The model under review builds one solid part; all positions refer to its coordinate system, in mm. A direction names the side the tool comes from. Give positions to 0.01 mm unless a question says otherwise; leave off trailing zeros. Loops run counter-clockwise (first coordinate to the right, second up) from the corner with the lowest first, then second, coordinate; pieces in that order, holes last. Notation, with made-up numbers: (89.5, -7) - (112.5, -7) arc R22 ccw to (112.5, 24) - close; hole circle Ø11 at (68.25, -27). An arc over 180 degrees is marked (long way). Answer as a JSON object with one key per item and string values.
from build123d import *

# Parameters (mm, degrees)
F0_R     = 26.9884014256
F1_DEPTH = 7
F2_R     = 32.0417466588
F2_R_2   = 26.9884014256
F3_DEPTH = 3
F4_R     = 11.1906834264
F5_DEPTH = 7
F6_R     = 4.0199304585
F7_DEPTH = 25
F9_DEPTH = 25
F10_SIZE = 5
F11_SIZE = 2


with BuildPart() as f1:
    # F0 (on Top) → F1 (new body)
    with BuildSketch(Plane.XY):
        Circle(F0_R)
    extrude(amount=F1_DEPTH)

    # F2 (on face) → F3 (join)
    with BuildSketch(Plane.XY.offset(7)):
        Circle(F2_R)
        Circle(F2_R_2, mode=Mode.SUBTRACT)
        Circle(F2_R_2)
    extrude(amount=F3_DEPTH)

    # F4 (on face) → F5 (cut)
    with BuildSketch(Plane.XY.offset(10)):
        Circle(F4_R)
    extrude(amount=-F5_DEPTH, mode=Mode.SUBTRACT)

    # F6 (on face) → F7 (cut)
    with BuildSketch(Plane.XY.offset(3)):
        Circle(F6_R)
    extrude(amount=-F7_DEPTH, mode=Mode.SUBTRACT)

    # F8 (on face) → F9 (cut)
    with BuildSketch(Plane.XY.offset(10)):
        with BuildLine():
            ThreePointArc((-15.0136980872, 1.4416950877), (-10.584772446, 10.7448688798), (-1.2161651409, 15.0336475058))
            Line((-1.2161651409, 15.0336475058), (-1.2161651409, 28.0388555672))
            ThreePointArc((-1.2161651409, 28.0388555672), (-19.7651192157, 19.9247720578), (-28.0281643074, 1.4416950877))
            Line((-28.0281643074, 1.4416950877), (-15.0136980872, 1.4416950877))
        make_face()
        with BuildLine():
            ThreePointArc((1.2975777549, 15.0268395529), (10.5846814228, 10.7449585461), (15.0056430278, 1.5232505708))
            Line((15.0056430278, 1.5232505708), (28.0238503219, 1.5232505708))
            ThreePointArc((28.0238503219, 1.5232505708), (19.7650570518, 19.9248337234), (1.2975777549, 28.0352059228))
            Line((1.2975777549, 28.0352059228), (1.2975777549, 15.0268395529))
        make_face()
        with BuildLine():
            ThreePointArc((15.0298348497, -1.262410143), (10.7403927, -10.5893144079), (1.4751854085, -15.0104444634))
            Line((1.4751854085, -15.0104444634), (1.4751854085, -28.0264215906))
            ThreePointArc((1.4751854085, -28.0264215906), (19.9202803133, -19.7696462135), (28.0368115127, -1.262410143))
            Line((28.0368115127, -1.262410143), (15.0298348497, -1.262410143))
        make_face()
        with BuildLine():
            ThreePointArc((-1.1481693356, -15.038993389), (-10.6271050963, -10.7030020205), (-15.0304418379, -1.2551625933))
            Line((-15.0304418379, -1.2551625933), (-28.0371369086, -1.2551625933))
            ThreePointArc((-28.0371369086, -1.2551625933), (-19.8072075166, -19.8829326197), (-1.1481693356, -28.0417222428))
            Line((-1.1481693356, -28.0417222428), (-1.1481693356, -15.038993389))
        make_face()
    extrude(amount=-F9_DEPTH, mode=Mode.SUBTRACT)

    # F10
    f10_edges = [f1.edges().sort_by_distance(p)[0] for p in [
        (-10.584772, 10.744869, 0),
        (10.584681, 10.744959, 0),
        (-10.627105, -10.703002, 0),
        (10.740393, -10.589314, 0),
    ]]
    chamfer(f10_edges, length=F10_SIZE)

    # F11
    f11_edges = [f1.edges().sort_by_distance(p)[0] for p in [
        (10.740393, -10.589314, 5),
        (-10.627105, -10.703002, 5),
        (10.584681, 10.744959, 5),
        (-10.584772, 10.744869, 5),
    ]]
    chamfer(f11_edges, length=F11_SIZE)


solid = f1.part
Q1. Consider section C-C, the plane z = 8.75. State the section outline as (x, y) points, plus the area to 3 significant figures.
Results:
{"outline": "circle Ø64.08 at (0, 0); hole (-28.04, -1.26) arc R28.07 ccw to (-1.15, -28.04) - (-1.15, -15.04) arc R15.08 cw to (-15.03, -1.26) - close; hole (-28.03, 1.44) - (-15.01, 1.44) arc R15.08 cw to (-1.22, 15.03) - (-1.22, 28.04) arc R28.07 ccw to start; hole circle Ø22.38 at (0, 0); hole (1.3, 15.03) arc R15.08 cw to (15.01, 1.52) - (28.02, 1.52) arc R28.07 ccw to (1.3, 28.04) - close; hole (1.48, -28.03) arc R28.07 ccw to (28.04, -1.26) - (15.03, -1.26) arc R15.08 cw to (1.48, -15.01) - close", "area": "1,210 mm^2"}
Q2. Clearance check with flat-ended pins moving along their axes: pin 1 Ø3 at (x, z) = (-11.5, 3.5) entering from +Y; pin 2 Ø1.5 at (x, z) = (-6.5, 8) entering from +Y; pin 3 Ø3 at (y, z) = (21, 6.5) entering from +X. State where each tip first meets the part, or that it passes through.
Results:
{"pin 1": "stops at y = 9.51", "pin 2": "stops at y = 31.52", "pin 3": "stops at x = 25.36"}
Q3. Consider section A-A, the plane y = 0. State the section outline as (x, z) points.
Results:
{"outline": "(-32.04, 7) - (-26.99, 7) - (-26.99, 0) - (-4.02, 0) - (-4.02, 3) - (-11.19, 3) - (-11.19, 10) - (-32.04, 10) - close; (4.02, 0) - (26.99, 0) - (26.99, 7) - (32.04, 7) - (32.04, 10) - (11.19, 10) - (11.19, 3) - (4.02, 3) - close"}
Q4. The part is to be moulded in two halves that separate along X. For faces 1 (the face through (26.99, 0.11, 3.45)), 2 (the face through (7, 10, 10)), 3 (the face through (-6.95, -31.28, 8.48)), 4 (the face through (1.298, 19, 5)), say which applies: +X half, -X half, draft (parallel to the pull), parting line (faces both ways), or undercut.
Results:
{"face 1": "+X half", "face 2": "draft", "face 3": "parting line", "face 4": "undercut"}
Q5. Consider section D-D, the plane x = 18.5. State the section outline as (y, z) points, plus the area to 3 significant figures.
Results:
{"outline": "(-26.16, 7) - (-21.1, 7) - (-21.1, 10) - (-26.16, 10) - close; (-1.26, 0) - (1.52, 0) - (1.52, 10) - (-1.26, 10) - close; (21.1, 7) - (26.16, 7) - (26.16, 10) - (21.1, 10) - close", "area": "58.2 mm^2"}
Q6. To check wall thickness, follow probe 1 along Y at (x, z) = (0, 6); probe 2 along Y at (x, z) = (0, 1.8); probe 3 along Y at (x, z) = (5.5, 7.75). State the ranges of each line that lie inside material, in increasing order. Write a range as [from, to].
Results:
{"probe 1": "y = [-26.99, -11.19], [11.19, 26.99]", "probe 2": "y = [-26.99, -4.02], [4.02, 26.99]", "probe 3": "y = [-31.57, -27.52], [-14.04, -9.75], [9.75, 14.04], [27.52, 31.57]"}
Q7. For faces 5 (the face through (-2.426, -10.925, 6.549)), 6 (the face through (-10.52, -10.81, 8.52)), 7 (the face through (1.475, -21, 5)), list the 3-axis set-ups (+Z, -Z, +X, -X, +Y, -Y) from which the entire face can be reached by the end or side of a thin tool; tool diameter is ignored.
Results:
{"face 5": "+Z", "face 6": "+Z, -Z", "face 7": "-Z"}
